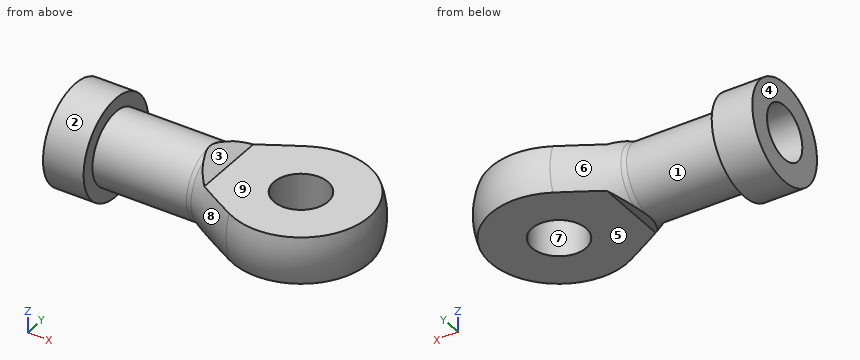
```python
from build123d import *

# Parameters (mm, degrees)
CUT_EXTRUDE_1_DEPTH = 17.5
SKETCH_3_R          = 6
CUT_EXTRUDE_2_DEPTH = 30
SKETCH_4_R          = 6
CUT_EXTRUDE_3_DEPTH = 30


with BuildPart() as part:
    # 草图1 → 旋转1 (revolve)
    with BuildSketch(Plane(origin=(0, 0, 0), x_dir=(1, 0, 0), z_dir=(0, 1, 0)), mode=Mode.PRIVATE) as revolve_1_sk:
        with BuildLine():
            Line((0, 0), (0, 11))
            Line((0, 11), (9, 11))
            Line((9, 11), (9, 8))
            Line((9, 8), (29.811328827, 8))
            ThreePointArc((29.811328827, 8), (30.38898409, 8.056139542), (30.945019819, 8.222457069))
            Line((30.945019819, 8.222457069), (42.711427769, 14.243479731))
            ThreePointArc((42.711427769, 14.243479731), (58.348138844, 13.649490021), (66, 0))
            Line((66, 0), (0, 0))
        make_face()
    revolve(revolve_1_sk.sketch.rotate(Axis((0, 0, 0), (1, 0, 0)), 180), axis=Axis((0, 0, 0), (1, 0, 0)))

    # 草图2 → 拉伸1 (cut, symmetric)
    with BuildSketch(Plane(origin=(0, 0, 0), x_dir=(1, 0, 0), z_dir=(0, 1, 0))):
        Polygon((72.287262903, 20.406671453), (73.576090576, 5.191308691), (34, 5.191308691), (29.811328827, 8), (29.00979021, 16.150849151), align=None)
        Polygon((34, -5.191308691), (29.811328827, -8), (29.00979021, -16.150849151), (72.287262903, -20.406671453), (73.576090576, -5.191308691), align=None)
    extrude(amount=CUT_EXTRUDE_1_DEPTH, both=True, mode=Mode.SUBTRACT)

    # 草图3 → 拉伸2 (cut)
    with BuildSketch(Plane(origin=(0, 0, -5.191308691), x_dir=(-1, 0, 0), z_dir=(0, 0, -1))):
        with Locations((-50, 0)):
            Circle(SKETCH_3_R)
    extrude(amount=-CUT_EXTRUDE_2_DEPTH, mode=Mode.SUBTRACT)

    # 草图4 → 拉伸3 (cut)
    with BuildSketch(Plane.ZY):
        Circle(SKETCH_4_R)
    extrude(amount=-CUT_EXTRUDE_3_DEPTH, mode=Mode.SUBTRACT)


solid = part.part
```
Here's how the part is built. I have some questions about the finished solid (model axes, mm). Face numbers are marked on the shaded views. A direction names the side the tool comes from. Round coordinates to 2 decimals unless told otherwise and drop trailing zeros. Loops run counter-clockwise (first coordinate to the right, second up) from the corner with the lowest first, then second, coordinate; pieces in that order, holes last.
1. Suppose I cut it at C-C, the plane x = 19.5. Please give me the cut outline in (y, z), and give its area (3 significant figures).
Answers:
outline: circle Ø16 at (0, 0); hole circle Ø12 at (0, 0)
area: 88.0 mm2
2. Suppose I cut it at B-B, the plane z = 0. Please give me the cut outline in (x, y).
Answers:
outline: (0, -11) - (9, -11) - (9, -8) - (29.81, -8) arc R3 cw to (30.95, -8.22) - (42.71, -14.24) arc R16 ccw (long way) to (42.71, 14.24) - (30.95, 8.22) arc R3 cw to (29.81, 8) - (9, 8) - (9, 11) - (0, 11) - (0, 6) - (30, 6) - (30, -6) - (0, -6) - close; hole circle Ø12 at (50, 0)
3. Will these pins go through, and if not, where does the flat tip stop? pin 1 (12 mm diameter, centred on y = 3, z = -2.5, fed in from +X); pin 2 (8 mm diameter, centred on x = 24.5, y = -8, fed in from -Z); pin 3 (5 mm diameter, centred on x = 58, z = -5, fed in from -Y); pin 4 (9 mm diameter, centred on x = 55.5, y = -1.5, fed in from -Z).
Answers:
pin 1: stops at x = 66
pin 2: stops at z = -6.93
pin 3: stops at y = -14.42
pin 4: stops at z = -5.19
4. For the marked faces 1, 2, 3, 4 and 5, which set-ups out of +Z, -Z, +X, -X, +Y, -Y let a thin tool reach every point of the face, with its end or its side?
Answers:
face 1: none
face 2: -X
face 3: +Z, +X, +Y, -Y
face 4: +Z, -Z, -X, +Y, -Y
face 5: -Z, +X, +Y, -Y
5. If I drill on probe 1 along Y at (x, z) = (12, 0); probe 2 along X at (y, z) = (-7.5, -5.5); probe 3 along Y at (x, z) = (19.5, 2), over which ranges is the centre line in solid material (lowest first)?
Answers:
probe 1: y = -8 to -6, 6 to 8
probe 2: x = 0 to 9, 33.05 to 33.54
probe 3: y = -7.75 to -5.66, 5.66 to 7.75
6. Suppose I cut it at D-D, the plane z = 9. Please give me the cut outline in (x, y), and give its area (3 significant figures).
Answers:
outline: (0, -6.32) - (9, -6.32) - (9, 6.32) - (0, 6.32) - close
area: 114 mm2
7. Suppose I cut it at A-A, the plane x = 50. Please give me the cut outline in (y, z).
Answers:
outline: (-15.13, -5.19) - (-6, -5.19) - (-6, 5.19) - (-15.13, 5.19) arc R16 ccw to start; (6, -5.19) - (15.13, -5.19) arc R16 ccw to (15.13, 5.19) - (6, 5.19) - close
8. Thinking about a two-plate mould opening in Y: for the marked faces 6, 7, 8 and 9, which applies, released by +Y, released by -Y, zero draft, split by the parting line, or undercut?
Answers:
face 6: released by +Y
face 7: undercut
face 8: released by -Y
face 9: zero draft
